For this review, use the dimensioned drawing (mm, ordinates from the lowest corner) and the shaded views. A direction names the side the tool comes from. Round coordinates to 2 decimals unless told otherwise and drop trailing zeros. Write each loop counter-clockwise with the first axis right and the second up, starting at its lowest first coordinate (ties: lowest second). Pieces come first, ordered by that corner, then holes. Notation, with made-up numbers: M -36,34 L 6,34 A29 cw 6,72 Z; hole C -37,9 d7. An arc over 180 degrees is marked long. Answer in a Markdown table with one row per item.
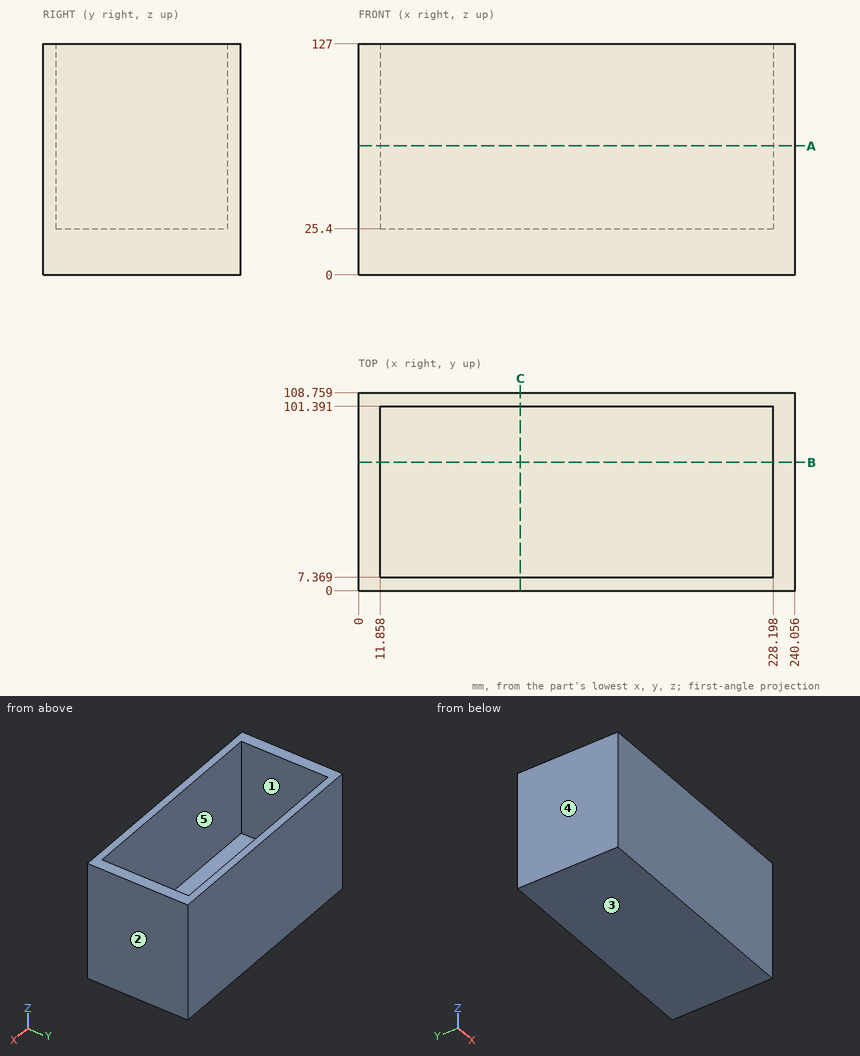
Q1. For probe 1 along X at (y, z) = (80, 117); probe 2 along Y at (x, z) = (138, 52); probe 3 along Z at (x, y) = (70, 84.5), list the stretches that pass through material, from the lowest coordinate up.
Found:
| item | result |
|---|---|
| probe 1 | 0 to 11.86, 228.2 to 240.06 |
| probe 2 | 0 to 7.37, 101.39 to 108.76 |
| probe 3 | 0 to 25.4 |
Q2. Take a section at C-C (x = 89). State the section outline as (y, z) points.
Found:
| item | result |
|---|---|
| outline | M 0,0 L 108.76,0 L 108.76,127 L 101.39,127 L 101.39,25.4 L 7.37,25.4 L 7.37,127 L 0,127 Z |
Q3. Take a section at B-B (y = 70.5). State the section outline as (x, z) points.
Found:
| item | result |
|---|---|
| outline | M 0,0 L 240.06,0 L 240.06,127 L 228.2,127 L 228.2,25.4 L 11.86,25.4 L 11.86,127 L 0,127 Z |
Q4. Machinability: for the marked faces 1 and 2, which of the approach directions +Z, -Z, +X, -X, +Y, -Y give a long, thin tool a straight path to every point of the face, cutting with its end or side? Answer none if there is none.
Found:
| item | result |
|---|---|
| face 1 | +Z |
| face 2 | +Z, -Z, +X, +Y, -Y |
Q5. Take a section at A-A (z = 71). State the section outline as (x, y) points.
Found:
| item | result |
|---|---|
| outline | M 0,0 L 240.06,0 L 240.06,108.76 L 0,108.76 Z; hole M 11.86,7.37 L 228.2,7.37 L 228.2,101.39 L 11.86,101.39 Z |
Q6. Mouldability with a two-part tool opening along X and no side actions: class the marked faces 3, 4 and 5 as +X half, -X half, draft (parallel to the pull), parting line (faces both ways), or undercut.
Found:
| item | result |
|---|---|
| face 3 | draft |
| face 4 | -X half |
| face 5 | undercut |
